Autodesk Inventor part; units mm, degrees
ref_plane "YZ Plane" through (0, 0, 0) normal (1, 0, 0) x (0, 1, 0)
ref_plane "XZ Plane" through (0, 0, 0) normal (0, 1, 0) x (-1, 0, 0)
ref_plane "XY Plane" through (0, 0, 0) normal (0, 0, 1) x (1, 0, 0)
sketch "Esquisse1" plane through (0, 0, 0) normal (0, 1, 0) x (-1, 0, 0)
  line L0 (-7.5, 7.5) -> (7.5, 7.5)
  line L1 (7.5, 7.5) -> (7.5, -7.5)
  line L2 (7.5, -7.5) -> (-7.5, -7.5)
  line L3 (-7.5, -7.5) -> (-7.5, 7.5)
  point P0 (0, 0)
  dimension "d0" = 15
  dimension "d1" = 15
  dimension "d2" = 7.5
  dimension "d3" = 7.5
extrude "Extrusion1" add sketch "Esquisse1" along normal blind 100
sketch "Esquisse2" plane through (0, 100, 0) normal (0, 1, 0) x (1, 0, 0)
  line L0 (-7.5, -7.5) -> (7.5, -7.5)
  line L1 (7.5, -7.5) -> (7.5, 7.5)
  line L2 (7.5, 7.5) -> (-7.5, 7.5)
  line L3 (-7.5, 7.5) -> (-7.5, -7.5)
  line L4 (-6.5, 6.5) -> (6.5, 6.5)
  line L5 (6.5, 6.5) -> (6.5, -6.5)
  line L6 (6.5, -6.5) -> (-6.5, -6.5)
  line L7 (-6.5, -6.5) -> (-6.5, 6.5)
  point P0 (0, 0)
  dimension "d6" = 1
  dimension "d7" = 1
  dimension "d8" = 1
  dimension "d9" = 1
extrude "Extrusion2" cut sketch "Esquisse2" against normal through all contours L4 L5 L6 L7
sketch "Esquisse3" plane through (7.5, 0, 7.5) normal (1, 0, 0) x (0, 0, -1)
  line L0 (15, 0) -> (0, 0)
  line L1 (15, 0) -> (15, 100)
  line L2 (0, 0) -> (0, 100)
  line L3 (1, 90) -> (14, 90)
  line L4 (14, 90) -> (14, 10)
  line L5 (14, 10) -> (1, 10)
  line L6 (1, 10) -> (1, 90)
  line L7 (1, 50) -> (14, 50) construction
  point P0 (7.5, 0)
  dimension "d12" = 80
  dimension "d13" = 1
  dimension "d14" = 1
  dimension "d15" = 100
  dimension "d16" = 50
extrude "Extrusion3" cut sketch "Esquisse3" against normal through all
sketch "Esquisse4" plane through (7.5, 0, 7.5) normal (1, 0, 0) x (0, 0, -1)
  line L0 (1, 10) -> (1, 90)
  line L1 (1, 90) -> (14, 90)
  line L2 (14, 90) -> (14, 10)
  line L3 (15, 0) -> (15, 100)
  line L4 (0, 0) -> (0, 100)
  line L5 (0, 90) -> (15, 90) construction
  line L6 (0, 90) -> (15, 100) construction
  line L7 (0, 100) -> (15, 90) construction
  circle A0 centre (7.5, 95) radius 3
  line L8 (1, 50) -> (14, 50) construction
  circle A1 centre (7.5, 5) radius 3
  point P0 (7.5, 0)
  dimension "d19" = 6
extrude "Extrusion4" cut sketch "Esquisse4" against normal through all
sketch "Esquisse5" plane through (7.5, 0, -7.5) normal (0, 0, -1) x (-1, 0, 0)
  line L0 (15, 0) -> (0, 0)
  line L1 (0, 100) -> (15, 100)
  line L2 (0, 0) -> (0, 100)
  circle A0 centre (7.5, 50) radius 3
  circle A1 centre (7.5, 40) radius 1.25
  circle A2 centre (7.5, 60) radius 1.25
  line L3 (7.5, 50) -> (0, 50) construction
  line L4 (7.5, 50) -> (7.5, 100) construction
  point P0 (7.5, 0)
  dimension "d22" = 6
  dimension "d23" = 100
  dimension "d24" = 50
  dimension "d25" = 7.5
  dimension "d26" = 10
  dimension "d27" = 2.5
extrude "Extrusion5" cut sketch "Esquisse5" against normal through all
equation "\"d16\" = 0.5 * d15"
properties part number "encoder_wheel_support"
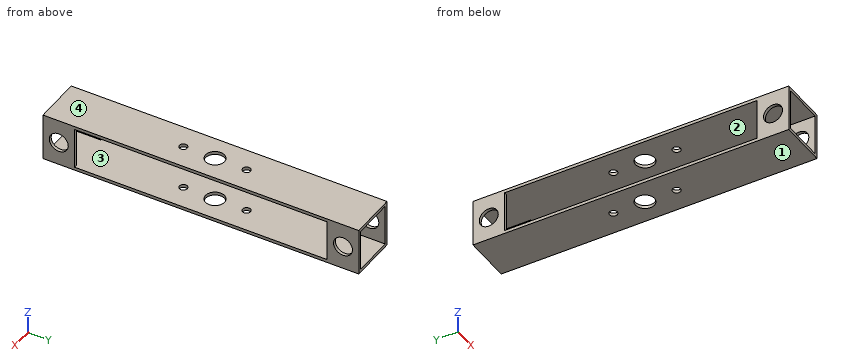
Could you check a few things on this model? Use its own coordinates, in mm. Face numbers are marked on the shaded views. A direction names the side the tool comes from. Give positions to 0.01 mm unless a question says otherwise; leave off trailing zeros. Order: outer loops, then holes, each group sorted by start corner. A loop starts at its lowest first (then second) coordinate and runs counter-clockwise, first axis right, second up.
Q1. Suppose I cut it at A-A, the plane y = 24.5. Write out the boundary of the cut face in (x, z), and give its area (3 significant figures).
Q2. Suppose I cut it at B-B, the plane z = -4. Write out the boundary of the cut face in (x, y).
Q3. Suppose I cut it at C-C, the plane x = 0. Count the separate pieces of the cut face and the enclosed holes in it, and give its area (3 significant figures).
Q4. We'd pull the mould along X, two halves only. Please class the marked faces 3 and 4: +X half, -X half, draft (parallel to the pull), parting line (faces both ways), or undercut.
Q5. For the marked faces 1 and 2, which set-ups out of +Z, -Z, +X, -X, +Y, -Y let a thin tool reach every point of the face, with its end or its side?
Q6. If I drill on line 1 along Y through (x, z) = (0, -6.9); line 2 along Y through (x, z) = (6.9, 0); line 3 along Z through (x, y) = (-1.5, 42), over which ranges is the centre line in solid material (lowest first)?
Q7. Suppose I cut it at D-D, the plane y = 60. Write out the boundary of the cut face in (x, z).
Solution:
1. outline: (-7.5, -7.5) - (7.5, -7.5) - (7.5, -6.5) - (-7.5, -6.5) - close; (-7.5, 6.5) - (7.5, 6.5) - (7.5, 7.5) - (-7.5, 7.5) - close
1. area: 30.0 mm2
2. outline: (-7.5, 0) - (-6.5, 0) - (-6.5, 10) - (-7.5, 10) - close; (-7.5, 90) - (-6.5, 90) - (-6.5, 100) - (-7.5, 100) - close; (6.5, 0) - (7.5, 0) - (7.5, 10) - (6.5, 10) - close; (6.5, 90) - (7.5, 90) - (7.5, 100) - (6.5, 100) - close
3. separate pieces: 8
3. enclosed holes: 0
3. area: 178 mm2
4. face 3: undercut
4. face 4: draft
5. face 1: -Z, +X, -X, +Y, -Y
5. face 2: none
6. line 1: y = 0 to 38.75, 41.25 to 47, 53 to 58.75, 61.25 to 100
6. line 2: y = 0 to 2, 8 to 10, 90 to 92, 98 to 100
6. line 3: z = -7.5 to -6.5, 6.5 to 7.5
7. outline: (-7.5, -7.5) - (-1.25, -7.5) - (-1.25, -6.5) - (-7.5, -6.5) - close; (-7.5, 6.5) - (-1.25, 6.5) - (-1.25, 7.5) - (-7.5, 7.5) - close; (1.25, -7.5) - (7.5, -7.5) - (7.5, -6.5) - (1.25, -6.5) - close; (1.25, 6.5) - (7.5, 6.5) - (7.5, 7.5) - (1.25, 7.5) - close
